Can you work these out from the model? Positions are in its coordinate system, mm. A direction names the side the tool comes from. Round coordinates to 2 decimals unless told otherwise and drop trailing zeros. Order: outer loops, then holes, each group sorted by start corner. A loop starts at its lowest first (then second) coordinate and runs counter-clockwise, first axis right, second up. Notation, with made-up numbers: M 83.5,-28 L 128.5,-28 A25 cw 128.5,-15 Z; hole C 89.25,79 d10. An arc over 180 degrees is marked long. Answer as a JSON object with one key per item and string values. Group by question number.
```python
from build123d import *

# Parameters (mm, degrees)
F0_W      = 50.8
F0_H      = 101.6
F1_DEPTH  = 1524
F2_W      = 50.8
F2_H      = 101.6
F3_DEPTH  = 914.4
F4_W      = 50.8
F4_H      = 101.6
F5_DEPTH  = 1524
F6_W      = 50.8
F6_H      = 101.6
F7_DEPTH  = 914.4
F8_W      = 50.8
F8_H      = 101.6
F9_DEPTH  = 1219.2
F10_W     = 50.8
F10_H     = 101.6
F11_DEPTH = 1219.2
F12_W     = 50.8
F12_H     = 101.6
F13_DEPTH = 609.6
F14_W     = 50.8
F14_H     = 101.6
F15_DEPTH = 609.6
F17_DEPTH = 101.6


with BuildPart() as f1:
    # F0 (on Front) → F1 (new body)
    with BuildSketch(Plane.XZ):
        with Locations((-25.4, 50.8)):
            Rectangle(F0_W, F0_H)
    extrude(amount=F1_DEPTH)

    # F2 (on Right) → F3 (join)
    with BuildSketch(Plane.YZ):
        with Locations((-25.4, 50.8)):
            Rectangle(F2_W, F2_H)
    extrude(amount=F3_DEPTH)

    # F4 (on face) → F5 (join)
    with BuildSketch(Plane(origin=(0, 0, 0), x_dir=(-1, 0, 0), z_dir=(0, 1, 0))):
        with Locations((-939.8, 50.8)):
            Rectangle(F4_W, F4_H)
    extrude(amount=-F5_DEPTH)

    # F6 (on face) → F7 (join)
    with BuildSketch(Plane.YZ):
        with Locations((-1498.6, 50.8)):
            Rectangle(F6_W, F6_H)
    extrude(amount=F7_DEPTH)

    # F8 (on face) → F9 (join)
    with BuildSketch(Plane.XY.offset(101.6)):
        with Locations((939.8, -1473.2)):
            Rectangle(F8_W, F8_H)
    extrude(amount=F9_DEPTH)

    # F10 (on face) → F11 (join)
    with BuildSketch(Plane.XY.offset(101.6)):
        with Locations((939.8, -50.8)):
            Rectangle(F10_W, F10_H)
    extrude(amount=F11_DEPTH)

    # F12 (on face) → F13 (join)
    with BuildSketch(Plane.XY.offset(101.6)):
        with Locations((-25.4, -50.8)):
            Rectangle(F12_W, F12_H)
    extrude(amount=F13_DEPTH)

    # F14 (on face) → F15 (join)
    with BuildSketch(Plane.XY.offset(101.6)):
        with Locations((-25.4, -1473.2)):
            Rectangle(F14_W, F14_H)
    extrude(amount=F15_DEPTH)

    # F16 (on face) → F17 (join)
    with BuildSketch(Plane.XZ.offset(1524)):
        Polygon((914.4, 1320.8), (-50.8, 711.2), (0, 711.2), (914.4, 1288.715789), align=None)
    extrude(amount=-F17_DEPTH)


solid = f1.part
```
1) If we section it at B-B on z = 869: Write out the boundary of the cut face in (x, y).
2) We'd pull the mould along Z, two halves only. Please class faces 1 (the face through (451, -1499, 101.6)), 2 (the face through (944, -822, 0)), 3 (the face through (939, -101.6, 703)): +Z half, -Z half, draft (parallel to the pull), parting line (faces both ways), or undercut.
3) I need wall thicknesses on line 1 along Z through (x, y) = (-2.5, -272); line 2 along Z through (x, y) = (13, -1456.5). Which ranges of each line are inside material? Lowest first, please.
4) Which directions (+Z, -Z, +X, -X, +Y, -Y) give clear straight access to the entire face, cutting with the end or side of a thin tool? Please do faces 4 (the face through (-26, -101.6, 402)), 5 (the face through (-26, -50, 711.2)), 6 (the face through (451, -26, 101.6)).
5) If we section it at C-C on y = -1224: Write out the boundary of the cut face in (x, z), plus the area to 3 significant figures.
6) For pin 1 (15 mm diameter, centred on x = -37, y = -53.5, fed in from +Z), with a flat end and sliding along its axis, tell me the tip position at first contact or that it passes through.
7) If we section it at D-D on x = 241: Write out the boundary of the cut face in (y, z).
8) If we section it at A-A on z = 221: Write out the boundary of the cut face in (x, y).
Findings:
{
 "1": {"outline": "M 199.05,-1524 L 249.85,-1524 L 249.85,-1422.4 L 199.05,-1422.4 Z; M 914.4,-1524 L 965.2,-1524 L 965.2,-1422.4 L 914.4,-1422.4 Z; M 914.4,-101.6 L 965.2,-101.6 L 965.2,0 L 914.4,0 Z"},
 "2": {"face 1": "undercut", "face 2": "-Z half", "face 3": "draft"},
 "3": {"line 1": "z = 0 to 101.6", "line 2": "z = 719.41 to 751.49"},
 "4": {"face 4": "+Z, +X, -X", "face 5": "+Z, -X, +Y", "face 6": "+Z, +Y, -Y"},
 "5": {"outline": "M -50.8,0 L 0,0 L 0,101.6 L -50.8,101.6 Z; M 914.4,0 L 965.2,0 L 965.2,101.6 L 914.4,101.6 Z", "area": "10,300 mm^2"},
 "6": {"pin 1": "stops at z = 711.2"},
 "7": {"outline": "M -1524,0 L -1473.2,0 L -1473.2,101.6 L -1524,101.6 Z; M -1524,863.41 L -1422.4,863.41 L -1422.4,895.49 L -1524,895.49 Z; M -50.8,0 L 0,0 L 0,101.6 L -50.8,101.6 Z"},
 "8": {"outline": "M -50.8,-1524 L 0,-1524 L 0,-1422.4 L -50.8,-1422.4 Z; M -50.8,-101.6 L 0,-101.6 L 0,0 L -50.8,0 Z; M 914.4,-1524 L 965.2,-1524 L 965.2,-1422.4 L 914.4,-1422.4 Z; M 914.4,-101.6 L 965.2,-101.6 L 965.2,0 L 914.4,0 Z"}
}
